```python
from build123d import *

# Parameters (mm, degrees)
F0_R          = 7.62
F1_DEPTH      = 25.4
F3_DEPTH      = 7.621
F3_DEPTH_BACK = 7.621
F4_R          = 1.27
F5_DEPTH      = 3.175


with BuildPart() as f1:
    # F0 (on Top) → F1 (new body)
    with BuildSketch(Plane.XY):
        Circle(F0_R)
    extrude(amount=F1_DEPTH)

    # F2 (on Front) → F3 (cut, two sides)
    with BuildSketch(Plane.XZ) as f3_sk:
        Polygon((-7.62, 36.5128359933), (-7.62, 13.3016251091), (-0.635, 25.4), (0, 26.4998522628), (0.635, 25.4), (7.62, 13.3016251091), (7.62, 36.5128359933), align=None)
        Polygon((0, 26.4998522628), (-0.635, 25.4), (0.635, 25.4), align=None)
    extrude(amount=-F3_DEPTH, mode=Mode.SUBTRACT)
    extrude(f3_sk.sketch, amount=F3_DEPTH_BACK, mode=Mode.SUBTRACT)

    # F4 (on face) → F5 (cut)
    with BuildSketch(Plane(origin=(0, 0, 0), x_dir=(1, 0, 0), z_dir=(0, 0, -1))):
        Circle(F4_R)
    extrude(amount=-F5_DEPTH, mode=Mode.SUBTRACT)


solid = f1.part
```
CAD build for the part. Positions are in the model's coordinates, mm. A direction names the side the tool comes from. Round coordinates to 2 decimals unless told otherwise and drop trailing zeros. Loops run counter-clockwise (first coordinate to the right, second up) from the corner with the lowest first, then second, coordinate; pieces in that order, holes last. Notation, with made-up numbers: M 49.5,42 L 54.5,42 A21 ccw 54.5,51 Z; hole C -11.75,-22 d9. An arc over 180 degrees is marked long. Return JSON: item names as keys, results as strings. Group by question number.
(1) Saw through at C-C, the plane z = 8.5. List the corners of the cut face in (x, y).
(2) Wall check: probe 1 along Y at (x, z) = (0, 0.9); probe 2 along Z at (x, y) = (0.25, -1) (3 decimals). Give the ranges that are in metal, low to high. Write a range as [from, to].
(3) Saw through at D-D, the plane y = 5.5. List the corners of the cut face in (x, z) (3 decimals), and give its area (3 significant figures).
(4) Saw through at A-A, the plane y = 0. List the corners of the cut face in (x, z) (3 decimals).
(5) Tool access for faces 1 (the flat face through (3.302, 0.106, 20.78)), 2 (the flat face through (0, 0, 3.175)): list every direction of +Z, -Z, +X, -X, +Y, -Y with a clear straight run to the whole face (end or side of a thin tool).
(6) Mould opens along X. For faces 3 (the cylindrical face through (-0.17, -1.26, 1.57)), 4 (the flat face through (-3.4, 0.11, 20.61)), 5 (the cylindrical face through (-5.616, 5.15, 9.7)) say: +X half, -X half, draft (parallel to the pull), parting line (faces both ways), or undercut.
(7) Saw through at B-B, the plane x = 0. List the corners of the cut face in (y, z) (3 decimals).
(8) Drop flat-ended pins along their axis: P1, Ø2, axis at x = -2, z = 8.5, coming from the +Y side; P2, Ø4, axis at x = -4.5, y = 3.5, coming from the +Z side; P3, Ø1.5, axis at x = 4, z = 13, coming from the +Y side. Give the stop position or say it passes through.
Answer list:
{
 "1": {"outline": "C 0,0 d15.24"},
 "2": {"probe 1": "[-7.62, -1.27], [1.27, 7.62]", "probe 2": "[3.175, 25.4]"},
 "3": {"outline": "M -5.274,0 L 5.274,0 L 5.274,17.365 L 0.635,25.4 L -0.635,25.4 L -5.274,17.365 Z", "area": "231 mm2"},
 "4": {"outline": "M -7.62,0 L -1.27,0 L -1.27,3.175 L 1.27,3.175 L 1.27,0 L 7.62,0 L 7.62,13.302 L 0.635,25.4 L -0.635,25.4 L -7.62,13.302 Z"},
 "5": {"face 1": "+Z, +X, +Y, -Y", "face 2": "-Z"},
 "6": {"face 3": "undercut", "face 4": "-X half", "face 5": "parting line"},
 "7": {"outline": "M -7.62,0 L -1.27,0 L -1.27,3.175 L 1.27,3.175 L 1.27,0 L 7.62,0 L 7.62,25.4 L -7.62,25.4 Z"},
 "8": {"P1": "y = 7.55", "P2": "z = 22.17", "P3": "y = 6.89"}
}
